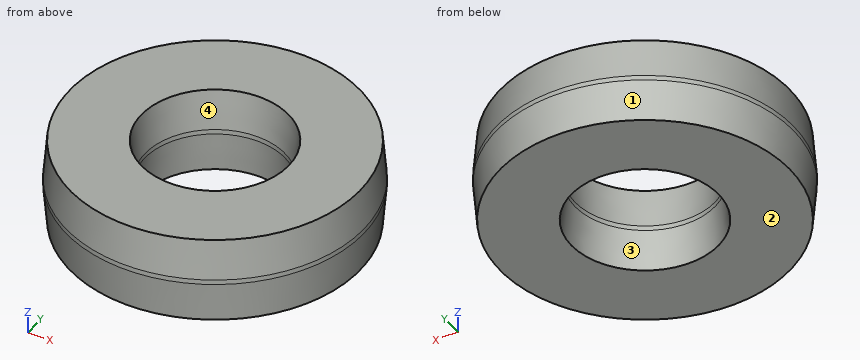
```python
from build123d import *

# Parameters (mm, degrees)
SKETCH_1_R      = 62.5
SKETCH_1_R_2    = 29.5
EXTRUDE_1_DEPTH = 17
EXTRUDE_1_DRAFT = 5
SKETCH_2_R      = 62.5
SKETCH_2_R_2    = 29.5
EXTRUDE_2_DEPTH = 2
SKETCH_3_R      = 62.5
SKETCH_3_R_2    = 29.5
EXTRUDE_3_DEPTH = 17
EXTRUDE_3_DRAFT = 5


with BuildPart() as part:
    # Эскиз1 → Вытянуть1 (with draft: the straight prism first)
    with BuildSketch(Plane.XY):
        Circle(SKETCH_1_R)
        Circle(SKETCH_1_R_2, mode=Mode.SUBTRACT)
    extrude(amount=EXTRUDE_1_DEPTH)
    # Вытянуть1: the draft: its side faces are tilted about the plane it starts from
    extrude_1_sides = [part.faces().sort_by_distance(p)[0] for p in [
        (-62.5, 0, 8.5),
        (-29.5, 0, 8.5),
    ]]
    draft(extrude_1_sides, Plane.XY, EXTRUDE_1_DRAFT)

    # Эскиз2 → Вытянуть2 (add)
    with BuildSketch(Plane(origin=(0, 0, 0), x_dir=(-1, 0, 0), z_dir=(0, 0, -1))):
        Circle(SKETCH_2_R)
        with Locations(Location((0, 0, 0), (0, 0, 180))):
            Circle(SKETCH_2_R_2, mode=Mode.SUBTRACT)
    extrude(amount=EXTRUDE_2_DEPTH)


with BuildPart() as extrude_3_tool:
    # Эскиз3 → Вытянуть3 (with draft: the straight prism first)
    with BuildSketch(Plane(origin=(0, 0, -2), x_dir=(-1, 0, 0), z_dir=(0, 0, -1))):
        Circle(SKETCH_3_R)
        with Locations(Location((0, 0, 0), (0, 0, 180))):
            Circle(SKETCH_3_R_2, mode=Mode.SUBTRACT)
    extrude(amount=EXTRUDE_3_DEPTH)
    # Вытянуть3: the draft: its side faces are tilted about the plane it starts from
    extrude_3_sides = [extrude_3_tool.faces().sort_by_distance(p)[0] for p in [
        (62.5, 0, -10.5),
        (-29.5, 0, -10.5),
    ]]
    draft(extrude_3_sides, Plane(origin=(0, 0, -2), x_dir=(-1, 0, 0), z_dir=(0, 0, -1)), EXTRUDE_3_DRAFT)


with BuildPart() as part_1:
    add(part.part)

    # Вытянуть3: add extrude_3_tool
    add(extrude_3_tool.part)


solid = part_1.part
```
Geometry: final body of the model. Coordinates: model frame, mm. Face numbers are marked on the shaded views. Round coordinates to 2 decimals unless told otherwise and drop trailing zeros. Order: outer loops, then holes, each group sorted by start corner. A loop starts at its lowest first (then second) coordinate and runs counter-clockwise, first axis right, second up. Notation, with made-up numbers: (65, 49.5) -> (78, 49.5) arc R18 cw to (78, 62.5) -> close; hole circle Ø10 at (-33.75, 32.5). An arc over 180 degrees is marked (long way). Use one line per item in the form item = value.
(1) Ray query, probe 1 along Y at (x, z) = (0, -1); probe 2 along X at (y, z) = (23, 9.5); probe 3 along Y at (x, z) = (18.5, 0). Return the intervals inside material, ascending. Write a range as [from, to].
Results list:
probe_1 = [-62.5, -29.5], [29.5, 62.5]
probe_2 = [-57.22, -19.77], [19.77, 57.22]
probe_3 = [-59.7, -22.98], [22.98, 59.7]
(2) Draft query along X for the marked faces 1, 2, 3 and 4. Return one class per face: pulls with the +X half, pulls with the -X half, needs draft (parallel to the pull), parting line crosses it, or undercut.
Results list:
face_1 = parting line crosses it
face_2 = needs draft
face_3 = undercut
face_4 = undercut
(3) Section C-C on z = -16. Return loops of the section in (x, y).
Results list:
outline = circle Ø122.55 at (0, 0); hole circle Ø61.45 at (0, 0)
(4) First-contact query: pin 1 Ø2 at (x, z) = (-17.5, -9) entering from -Y; pin 2 Ø12 at (x, z) = (49, 10) entering from -Y; pin 3 Ø3 at (x, z) = (-39.5, 6) entering from -Y. Flat tips, straight axial feed; report the tip coordinate or a pass-through.
Results list:
pin_1 = -59.66
pin_2 = -44.19
pin_3 = -48.97
(5) Section D-D on z = 6. Return loops of the section in (x, y).
Results list:
outline = circle Ø123.95 at (0, 0); hole circle Ø60.05 at (0, 0)
(6) Section A-A on x = 0. Return loops of the section in (y, z).
Results list:
outline = (-62.5, -2) -> (-61.01, -19) -> (-30.99, -19) -> (-29.5, -2) -> (-29.5, 0) -> (-30.99, 17) -> (-61.01, 17) -> (-62.5, 0) -> close; (29.5, -2) -> (30.99, -19) -> (61.01, -19) -> (62.5, -2) -> (62.5, 0) -> (61.01, 17) -> (30.99, 17) -> (29.5, 0) -> close
